For this review, take the finished solid that the model builds, in its own axes (mm). Coordinates: 2 decimals unless noted, no trailing zeros. Order: outer loops, then holes, each group sorted by start corner. A loop starts at its lowest first (then second) coordinate and runs counter-clockwise, first axis right, second up. Notation, with made-up numbers: M -16.75,10 L 38.25,10 A20 ccw 38.25,40 Z; hole C 85.25,9 d7. An arc over 180 degrees is marked long. Use one line per item in the form item = value. Start each with the question number.
```python
from build123d import *

# Parameters (mm, degrees)
F0_R     = 2.5527
F0_R_2   = 14.2875
F0_R_3   = 9.5504
F0_R_4   = 11.1125
F1_DEPTH = 6.35


with BuildPart() as f1:
    # F0 (on Front) → F1 (new body)
    with BuildSketch(Plane.XZ):
        with BuildLine():
            Line((-99.456923, 38.339287), (-45.021703, -19.243367))
            ThreePointArc((-45.021703, -19.243367), (-42.050874, -21.366962), (-38.499317, -22.216626))
            Line((-38.499317, -22.216626), (-0.931741, -23.792961))
            ThreePointArc((-0.931741, -23.792961), (0, -23.8125), (0.931741, -23.792961))
            Line((0.931741, -23.792961), (38.499317, -22.216626))
            ThreePointArc((38.499317, -22.216626), (42.050874, -21.366962), (45.021703, -19.243367))
            Line((45.021703, -19.243367), (99.456923, 38.339287))
            ThreePointArc((99.456923, 38.339287), (108.045638, 63.504837), (94.65047, 86.475261))
            Line((94.65047, 86.475261), (68.686167, 104.794528))
            ThreePointArc((68.686167, 104.794528), (63.4647, 107.386922), (57.703744, 108.278896))
            Line((57.703744, 108.278896), (-57.703744, 108.278896))
            ThreePointArc((-57.703744, 108.278896), (-63.4647, 107.386922), (-68.686167, 104.794528))
            Line((-68.686167, 104.794528), (-94.65047, 86.475261))
            ThreePointArc((-94.65047, 86.475261), (-108.045638, 63.504837), (-99.456923, 38.339287))
        make_face()
        with Locations((-38.1, -12.7)):
            Circle(F0_R, mode=Mode.SUBTRACT)
        with Locations((-53.975, -1.5875)):
            Circle(F0_R, mode=Mode.SUBTRACT)
        with Locations((0, -1.5875)):
            Circle(F0_R_2, mode=Mode.SUBTRACT)
        with Locations((-38.1, 12.7)):
            Circle(F0_R, mode=Mode.SUBTRACT)
        with Locations((-31.75, 31.4325)):
            Circle(F0_R, mode=Mode.SUBTRACT)
        with Locations((38.1, -12.7)):
            Circle(F0_R, mode=Mode.SUBTRACT)
        with Locations((53.975, -1.5875)):
            Circle(F0_R, mode=Mode.SUBTRACT)
        with Locations((38.1, 12.7)):
            Circle(F0_R, mode=Mode.SUBTRACT)
        with Locations((31.75, 31.4325)):
            Circle(F0_R, mode=Mode.SUBTRACT)
        with Locations((-99.220218, 49.590496)):
            Circle(F0_R, mode=Mode.SUBTRACT)
        with Locations((-76.2, 60.325)):
            Circle(F0_R_3, mode=Mode.SUBTRACT)
        with Locations((-49.937819, 50.751531)):
            Circle(F0_R_4, mode=Mode.SUBTRACT)
        with Locations((-53.179782, 71.059504)):
            Circle(F0_R, mode=Mode.SUBTRACT)
        with Locations((0, 69.5325)):
            Circle(F0_R_2, mode=Mode.SUBTRACT)
        with Locations((-57.703744, 89.228896)):
            Circle(F0_R_4, mode=Mode.SUBTRACT)
        with Locations((-26.9875, 101.928896)):
            Circle(F0_R, mode=Mode.SUBTRACT)
        with Locations((49.937819, 50.751531)):
            Circle(F0_R_4, mode=Mode.SUBTRACT)
        with Locations((53.179782, 71.059504)):
            Circle(F0_R, mode=Mode.SUBTRACT)
        with Locations((99.220218, 49.590496)):
            Circle(F0_R, mode=Mode.SUBTRACT)
        with Locations((76.2, 60.325)):
            Circle(F0_R_3, mode=Mode.SUBTRACT)
        with Locations((26.9875, 101.928896)):
            Circle(F0_R, mode=Mode.SUBTRACT)
        with Locations((57.703744, 89.228896)):
            Circle(F0_R_4, mode=Mode.SUBTRACT)
    extrude(amount=F1_DEPTH)


solid = f1.part
```
1. The part is to be moulded in two halves that separate along X. For faces 1 (the flat face through (-2, 0, 43)), 2 (the cylindrical face through (-42.098, -3.131, -21.345)), 3 (the cylindrical face through (-58.756, -3.131, 43.99)), say which applies: pulls with the +X half, pulls with the -X half, needs draft (parallel to the pull), parting line crosses it, or undercut.
2. For pin 1 Ø17 at (x, z) = (0, -1.59) entering from +Y; pin 2 Ø2 at (x, y) = (63.5, -2.5) entering from -Z; pin 3 Ø1.5 at (x, y) = (6, -2.5) entering from -Z; pin 4 Ø1.5 at (y, z) = (-3.5, -4) entering from -X, all flat-tipped, find the tip position at first contact; note any pin that passes through.
3. Consider section B-B, the plane z = -12.7. Write out the cut boundary in (x, y), plus the area to 3 significant figures.
4. Consider section C-C, the plane y = -3.75. Give the number of separate pieces and of enclosed holes in the cut face, plus the area to 3 significant figures.
5. Consider section A-A, the plane x = -80.5. Write out the cut boundary in (y, z).
6. Consider section D-D, the plane x = -31.75. Write out the cut boundary in (y, z).
7. To check wall thickness, follow line 1 (Z direction, x = -4.5, y = -5); line 2 (X direction, y = -1.75, z = 33.5); line 3 (X direction, y = -4.5, z = 92). State the ranges of each line that lie inside material, in increasing order.
Answers follow:
q1.face_1 = needs draft
q1.face_2 = pulls with the -X half
q1.face_3 = undercut
q2.pin_1 = through
q2.pin_2 = -0.75
q2.pin_3 = -23.61
q2.pin_4 = -60.14
q3.outline = M -51.21,-6.35 L -40.65,-6.35 L -40.65,0 L -51.21,0 Z; M -35.55,-6.35 L -8.98,-6.35 L -8.98,0 L -35.55,0 Z; M 8.98,-6.35 L 35.55,-6.35 L 35.55,0 L 8.98,0 Z; M 40.65,-6.35 L 51.21,-6.35 L 51.21,0 L 40.65,0 Z
q3.area = 471 mm²
q4.separate_pieces = 1
q4.enclosed_holes = 22
q4.area = 18,500 mm²
q5.outline = M -6.35,18.29 L 0,18.29 L 0,51.8 L -6.35,51.8 Z; M -6.35,68.85 L 0,68.85 L 0,96.46 L -6.35,96.46 Z
q6.outline = M -6.35,-22.5 L 0,-22.5 L 0,28.88 L -6.35,28.88 Z; M -6.35,33.99 L 0,33.99 L 0,108.28 L -6.35,108.28 Z
q7.line_1 = -23.64 to -15.15, 11.97 to 55.97, 83.09 to 108.28
q7.line_2 = -94.88 to -33.25, -30.25 to 30.25, 33.25 to 94.88
q7.line_3 = -86.82 to -68.47, -46.94 to 46.94, 68.47 to 86.82
